Here's the drawing with two shaded views (mm, measured from the low corner). I have some questions. A direction names the side the tool comes from. Give positions to 0.01 mm unless a question says otherwise; leave off trailing zeros. Loops run counter-clockwise (first coordinate to the right, second up) from the corner with the lowest first, then second, coordinate; pieces in that order, holes last. Notation, with made-up numbers: (-18.75, -31.75) -> (10.25, -31.75) arc R20 ccw to (10.25, 6.25) -> close; hole circle Ø4 at (81.5, 82.5). An arc over 180 degrees is marked (long way). Answer in a Markdown table with one row per item. Add a question column.
Item 1: If we section it at C-C (y = 28): Write out the boundary of the cut face in (x, z).
Item 2: Which directions (+Z, -Z, +X, -X, +Y, -Y) give clear straight access to the entire face, cutting with the end or side of a thin tool? Please do the marked faces 1, 2 and 3.
Item 3: If we section it at D-D (z = 2.8): Write out the boundary of the cut face in (x, y), then the cut area to 3 significant figures.
Item 4: If I drill on line 1 (Z direction, x = 29.5, y = 29); line 2 (X direction, y = 3.15, z = 7.5); line 3 (X direction, y = 27.5, z = 4), over which ranges is the centre line in solid material (lowest first)?
Item 5: If we section it at B-B (x = 29.5): Write out the boundary of the cut face in (y, z).
Item 6: For P1, Ø3.5, axis at y = 28.83, z = 2.8, coming from the -X side; P2, Ø5, axis at x = 3.5, z = 13.5, coming from the -Y side; P3, Ø3, axis at x = 11.5, z = 7, coming from the +Y side; P4, Ø2, axis at x = 25, z = 8.5, coming from the +Y side, each with a flat end and sliding along its axis, tell me the tip position at first contact or that it passes through.
Item 7: If we section it at A-A (z = 7.5): Write out the boundary of the cut face in (x, y), then the cut area to 3 significant figures.
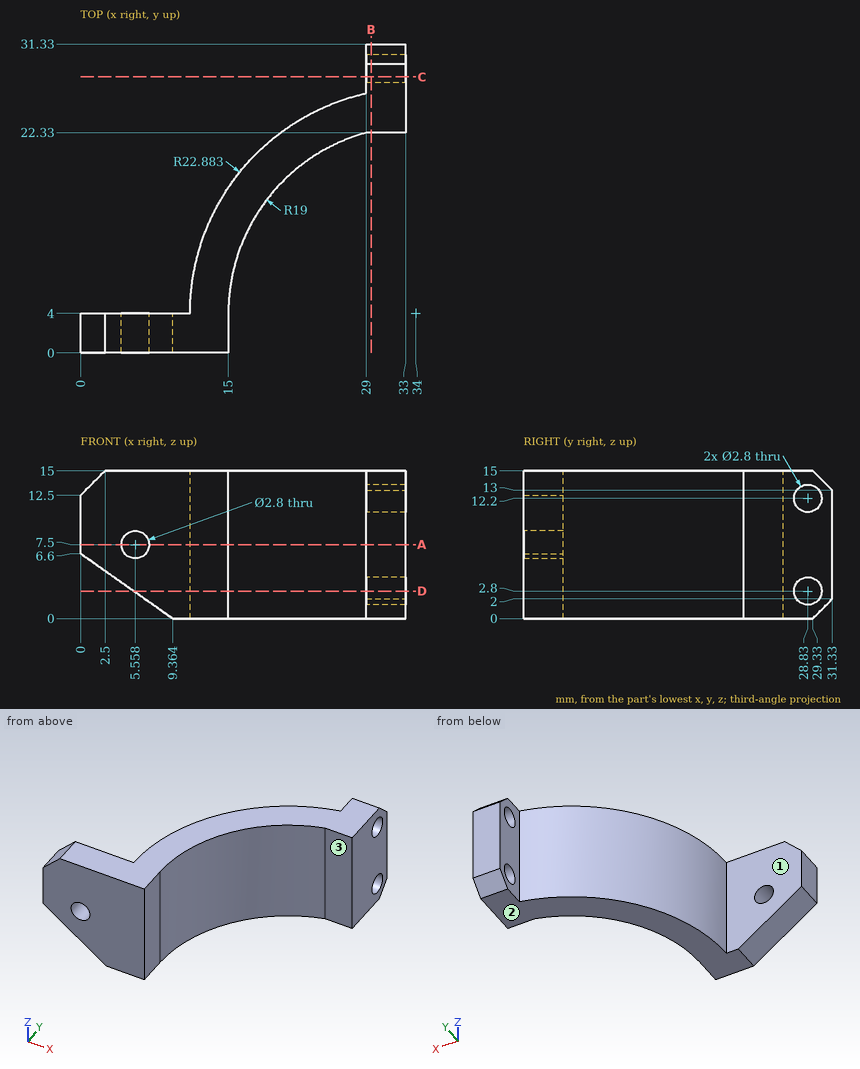
Recorded:
| question | item | result |
|---|---|---|
| 1 | outline | (29, 0) -> (33, 0) -> (33, 1.67) -> (29, 1.67) -> close; (29, 3.93) -> (33, 3.93) -> (33, 11.07) -> (29, 11.07) -> close; (29, 13.33) -> (33, 13.33) -> (33, 15) -> (29, 15) -> close |
| 2 | face 1 | +Z, -Z, -X, +Y |
| 2 | face 2 | -Z, +X, -X, +Y, -Y |
| 2 | face 3 | +Z, -Z, +X, -Y |
| 3 | outline | (5.39, 0) -> (15, 0) -> (15, 4) arc R19 cw to (29, 22.33) -> (33, 22.33) -> (33, 27.43) -> (29, 27.43) -> (29, 26.33) arc R22.88 ccw to (11.12, 4) -> (5.39, 4) -> close; (29, 30.23) -> (33, 30.23) -> (33, 31.33) -> (29, 31.33) -> close |
| 3 | area | 171 mm^2 |
| 4 | line 1 | z = 0 to 1.41, 4.19 to 10.81, 13.59 to 15 |
| 4 | line 2 | x = 0 to 4.16, 6.96 to 15 |
| 4 | line 3 | x = 29 to 33 |
| 5 | outline | (22.33, 0) -> (29.33, 0) -> (31.33, 2) -> (31.33, 13) -> (29.33, 15) -> (22.33, 15) -> close; hole circle Ø2.8 at (28.83, 2.8); hole circle Ø2.8 at (28.83, 12.2) |
| 6 | P1 | stops at x = 29 |
| 6 | P2 | stops at y = 0 |
| 6 | P3 | stops at y = 13.09 |
| 6 | P4 | stops at y = 25.44 |
| 7 | outline | (0, 0) -> (4.16, 0) -> (4.16, 4) -> (0, 4) -> close; (6.96, 0) -> (15, 0) -> (15, 4) arc R19 cw to (29, 22.33) -> (33, 22.33) -> (33, 31.33) -> (29, 31.33) -> (29, 26.33) arc R22.88 ccw to (11.12, 4) -> (6.96, 4) -> close |
| 7 | area | 193 mm^2 |
